Here's the drawing with two shaded views (mm, measured from the low corner). I have some questions. Coordinates: 2 decimals unless noted, no trailing zeros. Write each loop counter-clockwise with the first axis right and the second up, starting at its lowest first coordinate (ties: lowest second). Pieces come first, ordered by that corner, then holes.
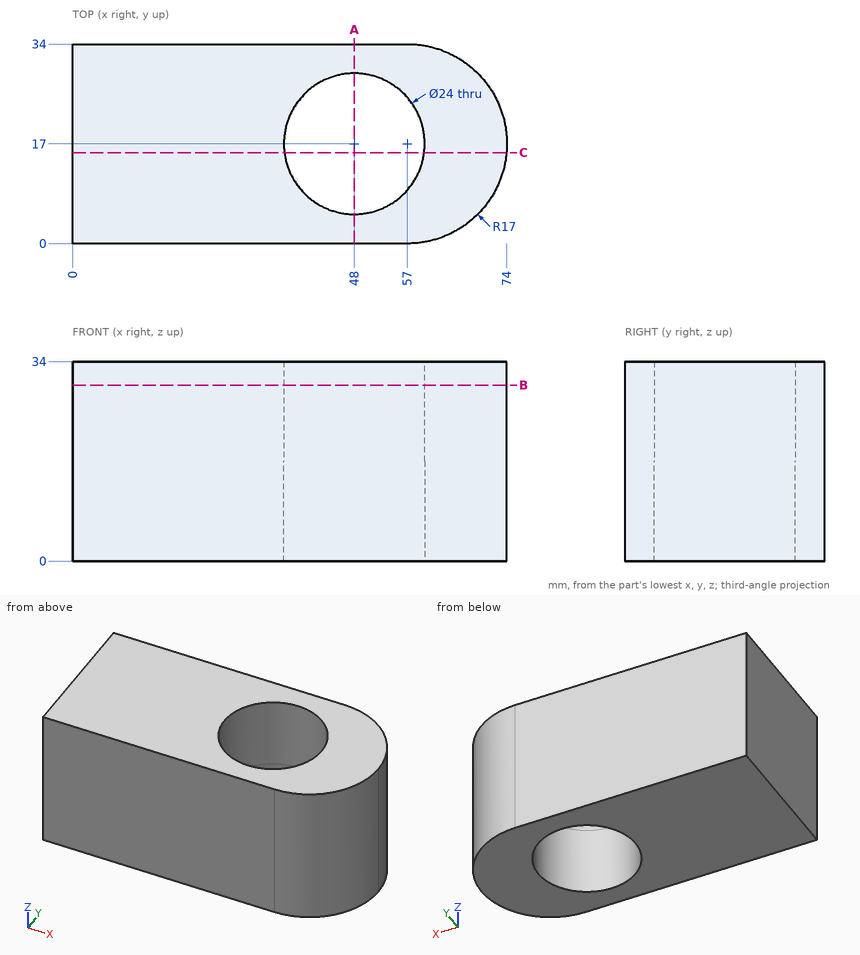
1. If we section it at C-C, the plane y = 15.5: List the corners of the cut face in (x, z) for me, plus the area to 3 significant figures.
2. I'm going to push flat-ended pins straight in: P1, Ø3, axis at y = 20.5, z = 16.5, coming from the +X side; P2, Ø2, axis at x = 59, z = 6, coming from the -Y side. Where does each tip first touch, or does it pass through?
3. If we section it at B-B, the plane z = 30: List the corners of the cut face in (x, y) for me.
4. If we section it at A-A, the plane x = 48: List the corners of the cut face in (y, z) for me, plus the area to 3 significant figures.
5. If I drill on L1, parallel to Y at x = 48, z = 7; L2, parallel to X at y = 10.5, z = 18; L3, parallel to X at y = 27, z = 20.5, over which ranges is the centre line in solid material (lowest first)?
Answers:
1. outline: (0, 0) - (36.09, 0) - (36.09, 34) - (0, 34) - close; (59.91, 0) - (73.93, 0) - (73.93, 34) - (59.91, 34) - close
1. area: 1,700 mm2
2. P1: stops at x = 73.88
2. P2: stops at y = 0.03
3. outline: (0, 0) - (57, 0) arc R17 ccw to (57, 34) - (0, 34) - close; hole circle Ø24 at (48, 17)
4. outline: (0, 0) - (5, 0) - (5, 34) - (0, 34) - close; (29, 0) - (34, 0) - (34, 34) - (29, 34) - close
4. area: 340 mm2
5. L1: y = 0 to 5, 29 to 34
5. L2: x = 0 to 37.91, 58.09 to 72.71
5. L3: x = 0 to 41.37, 54.63 to 70.75
